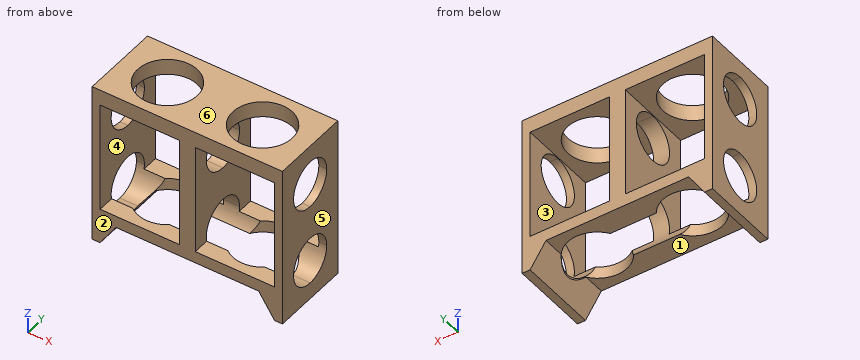
```python
from build123d import *

# Parameters (mm, degrees)
F0_W     = 20
F0_H     = 28
F1_DEPTH = 20
F3_DEPTH = 50
F5_DEPTH = 50


with BuildPart() as f1:
    # F0 (on Front) → F1 (new body)
    with BuildSketch(Plane.XZ):
        Polygon((0, 3), (0, 0), (18, 0), (22, -6), (24, -6), (24, 35), (22, 35), (0, 35), align=None)
        with Locations((12, 17)):
            Rectangle(F0_W, F0_H, mode=Mode.SUBTRACT)
        Polygon((-18, 0), (0, 0), (0, 3), (0, 35), (-22, 35), (-24, 35), (-24, -6), (-22, -6), align=None)
        with Locations((-12, 17)):
            Rectangle(F0_W, F0_H, mode=Mode.SUBTRACT)
    extrude(amount=F1_DEPTH)

    # F2 (on face) → F3 (cut)
    with BuildSketch(Plane.XY.offset(35)):
        with BuildLine():
            ThreePointArc((-19.5, -10), (-12, -17.5), (-4.5, -10))
            Line((-4.5, -10), (-19.5, -10))
        make_face()
        with BuildLine():
            Line((-19.5, -10), (-4.5, -10))
            ThreePointArc((-4.5, -10), (-12, -2.5), (-19.5, -10))
        make_face()
        with BuildLine():
            Line((19.5, -10), (4.5, -10))
            ThreePointArc((4.5, -10), (12, -17.5), (19.5, -10))
        make_face()
        with BuildLine():
            ThreePointArc((19.5, -10), (12, -2.5), (4.5, -10))
            Line((4.5, -10), (19.5, -10))
        make_face()
    extrude(amount=-F3_DEPTH, mode=Mode.SUBTRACT)

    # F4 (on face) → F5 (cut)
    with BuildSketch(Plane.YZ.offset(24)):
        with BuildLine():
            ThreePointArc((-10, 30.75), (-16, 24.75), (-10, 18.75))
            Line((-10, 18.75), (-10, 30.75))
        make_face()
        with BuildLine():
            Line((-10, 30.75), (-10, 18.75))
            ThreePointArc((-10, 18.75), (-5.7573593129, 20.5073593129), (-4, 24.75))
            ThreePointArc((-4, 24.75), (-5.7573593129, 28.9926406871), (-10, 30.75))
        make_face()
        with BuildLine():
            Line((-10, 10.25), (-10, -1.75))
            ThreePointArc((-10, -1.75), (-5.7573593129, 0.0073593129), (-4, 4.25))
            ThreePointArc((-4, 4.25), (-5.7573593129, 8.4926406871), (-10, 10.25))
        make_face()
        with BuildLine():
            ThreePointArc((-10, 10.25), (-16, 4.25), (-10, -1.75))
            Line((-10, -1.75), (-10, 10.25))
        make_face()
    extrude(amount=-F5_DEPTH, mode=Mode.SUBTRACT)


solid = f1.part
```
Can you work these out from the model? Positions are in its coordinate system, mm. Face numbers are marked on the shaded views. A direction names the side the tool comes from. Coordinates: 2 decimals unless noted, no trailing zeros. Order: outer loops, then holes, each group sorted by start corner. A loop starts at its lowest first (then second) coordinate and runs counter-clockwise, first axis right, second up. Notation, with made-up numbers: (-2, -35.75) - (42, -35.75) arc R7 cw to (42, -27.75) - close; hole circle Ø1 at (8.5, 5.5). An arc over 180 degrees is marked (long way). Answer in a Markdown table with one row per item.
1. For pin 1 (3 mm diameter, centred on x = 7.5, y = -15, fed in from -Z); pin 2 (6 mm diameter, centred on x = -16.5, y = -5.5, fed in from -Z), each with a flat end and sliding along its axis, tell me the tip position at first contact or that it passes through.
Reply:
| item | result |
|---|---|
| pin 1 | stops at z = 0 |
| pin 2 | stops at z = -2.25 |
2. If we mould it in two halves opening along X, with no side actions, what happens to the marked faces 4, 5 and 6? For each: pulls with the +X half, pulls with the -X half, needs draft (parallel to the pull), parting line crosses it, or undercut.
Reply:
| item | result |
|---|---|
| face 4 | undercut |
| face 5 | pulls with the +X half |
| face 6 | needs draft |
3. Suppose I cut it at B-B (z = 8.5). Please give me the cut outline in (x, y), and give its area (3 significant figures).
Reply:
| item | result |
|---|---|
| outline | (-24, -20) - (-22, -20) - (-22, -14.24) - (-24, -14.24) - close; (-24, -5.76) - (-22, -5.76) - (-22, 0) - (-24, 0) - close; (-2, -20) - (2, -20) - (2, -14.24) - (-2, -14.24) - close; (-2, -5.76) - (2, -5.76) - (2, 0) - (-2, 0) - close; (22, -20) - (24, -20) - (24, -14.24) - (22, -14.24) - close; (22, -5.76) - (24, -5.76) - (24, 0) - (22, 0) - close |
| area | 92.2 mm^2 |
4. For the marked faces 1, 2 and 3, which set-ups out of +Z, -Z, +X, -X, +Y, -Y let a thin tool reach every point of the face, with its end or its side?
Reply:
| item | result |
|---|---|
| face 1 | -Z, +Y, -Y |
| face 2 | +Z, -Z, +X, -X, -Y |
| face 3 | +Y, -Y |
5. If I drill on line 1 along X through (y, z) = (-10.5, 13); line 2 along Z through (x, y) = (-17.5, -2.75); line 3 along Y through (x, z) = (12, 1.6), over which ranges is the centre line in solid material (lowest first)?
Reply:
| item | result |
|---|---|
| line 1 | x = -24 to -22, -2 to 2, 22 to 24 |
| line 2 | z = 0 to 3, 31 to 35 |
| line 3 | y = -20 to -17.5, -2.5 to 0 |
6. Suppose I cut it at D-D (x = 3). Please give me the cut outline in (y, z), and give its area (3 significant figures).
Reply:
| item | result |
|---|---|
| outline | (-20, 0) - (-14.24, 0) arc R6 cw to (-15.87, 3) - (-20, 3) - close; (-20, 31) - (0, 31) - (0, 35) - (-20, 35) - close; (-5.76, 0) - (0, 0) - (0, 3) - (-4.13, 3) arc R6 cw to start |
| area | 109 mm^2 |
7. Suppose I cut it at C-C (x = -21). Please give me the cut outline in (y, z), and give its area (3 significant figures).
Reply:
| item | result |
|---|---|
| outline | (-20, -4.5) - (0, -4.5) - (0, 3) - (-4.13, 3) arc R6 cw to (-15.87, 3) - (-20, 3) - close; (-20, 31) - (0, 31) - (0, 35) - (-20, 35) - close |
| area | 188 mm^2 |
8. Suppose I cut it at A-A (x = 12). Please give me the cut outline in (y, z).
Reply:
| item | result |
|---|---|
| outline | (-20, 0) - (-17.5, 0) - (-17.5, 3) - (-20, 3) - close; (-20, 31) - (-17.5, 31) - (-17.5, 35) - (-20, 35) - close; (-2.5, 0) - (0, 0) - (0, 3) - (-2.5, 3) - close; (-2.5, 31) - (0, 31) - (0, 35) - (-2.5, 35) - close |
